For this review, use the dimensioned drawing (mm, ordinates from the lowest corner) and the shaded views. A direction names the side the tool comes from. Give positions to 0.01 mm unless a question says otherwise; leave off trailing zeros. Write each loop counter-clockwise with the first axis right and the second up, starting at its lowest first coordinate (ties: lowest second). Pieces come first, ordered by that corner, then holes. Notation, with made-up numbers: (14, 87.5) -> (32, 87.5) arc R17 ccw to (32, 92.5) -> close; hole circle Ø7 at (8, 63). An arc over 180 degrees is marked (long way). Return JSON: item names as keys, results as strings.
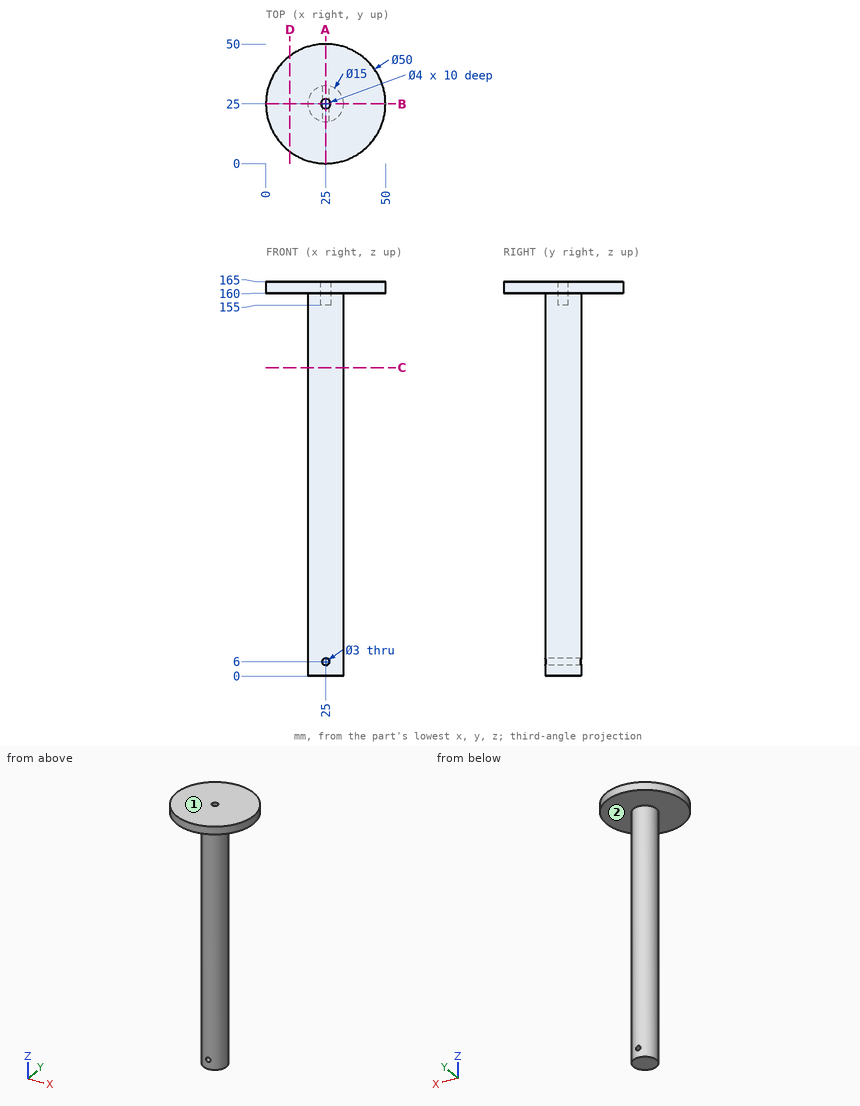
1. For pin 1 (2.5 mm diameter, centred on x = 25, z = 6, fed in from -Y); pin 2 (10 mm diameter, centred on y = 18.5, z = 142.5, fed in from +X); pin 3 (6 mm diameter, centred on x = 37.5, y = 9, fed in from -Z); pin 4 (3 mm diameter, centred on y = 25.5, z = 57.5, fed in from +X), all flat-tipped, find the tip position at first contact; note any pin that passes through.
Results found:
{"pin 1": "passes through", "pin 2": "stops at x = 32.35", "pin 3": "stops at z = 160", "pin 4": "stops at x = 32.5"}
2. Add section D-D, the plane x = 10. State the section outline as (y, z) points.
Results found:
{"outline": "(5, 160) -> (45, 160) -> (45, 165) -> (5, 165) -> close"}
3. Add section A-A, the plane x = 25. State the section outline as (y, z) points.
Results found:
{"outline": "(0, 160) -> (17.5, 160) -> (17.5, 7.5) -> (32.5, 7.5) -> (32.5, 160) -> (50, 160) -> (50, 165) -> (27, 165) -> (27, 155) -> (23, 155) -> (23, 165) -> (0, 165) -> close; (17.5, 0) -> (32.5, 0) -> (32.5, 4.5) -> (17.5, 4.5) -> close"}
4. To check wall thickness, follow probe 1 along Z at (x, y) = (25, 29.25); probe 2 along Y at (x, z) = (25, 157.75); probe 3 along Z at (x, y) = (8.5, 16). State the ranges of each line that lie inside material, in increasing order.
Results found:
{"probe 1": "z = 0 to 4.5, 7.5 to 165", "probe 2": "y = 17.5 to 23, 27 to 32.5", "probe 3": "z = 160 to 165"}
5. Add section B-B, the plane y = 25. State the section outline as (x, z) points, plus the area to 3 significant figures.
Results found:
{"outline": "(0, 160) -> (17.5, 160) -> (17.5, 0) -> (32.5, 0) -> (32.5, 160) -> (50, 160) -> (50, 165) -> (27, 165) -> (27, 155) -> (23, 155) -> (23, 165) -> (0, 165) -> close; hole circle Ø3 at (25, 6)", "area": "2,600 mm²"}
6. Add section C-C, the plane z = 129. State the section outline as (x, y) points, plus the area to 3 significant figures.
Results found:
{"outline": "circle Ø15 at (25, 25)", "area": "177 mm²"}
7. For the marked faces 1 and 2, list the 3-axis set-ups (+Z, -Z, +X, -X, +Y, -Y) from which the entire face can be reached by the end or side of a thin tool; tool diameter is ignored.
Results found:
{"face 1": "+Z, +X, -X, +Y, -Y", "face 2": "-Z"}
